```python
from build123d import *

# Parameters (mm, degrees)
F0_W     = 31.75
F0_H     = 88.9
F1_DEPTH = 2.54
F2_W     = 27.860178
F2_H     = 10.831637
F3_DEPTH = 25.4
F4_R     = 9.525
F5_DEPTH = 76.2
F6_R     = 7.62


with BuildPart() as f1:
    # F0 (on Top) → F1 (new body)
    with BuildSketch(Plane.XY):
        Rectangle(F0_W, F0_H)
    extrude(amount=F1_DEPTH)

    # F2 (on face) → F3 (join)
    with BuildSketch(Plane.XY.offset(2.54)):
        Polygon((15.875, -44.45), (15.875, 44.45), (14.305094, 44.45), (14.305094, -24.071639), (-13.428997, -24.071639), (-13.428997, 44.45), (-15.643887, 44.45), (-15.875, 44.45), (-15.875, -44.45), align=None)
        with Locations((0.375005, -33.933696)):
            Rectangle(F2_W, F2_H, mode=Mode.SUBTRACT)
    extrude(amount=F3_DEPTH)

    # F4 (on face) → F5 (join)
    with BuildSketch(Plane(origin=(0, -24.071639, 0), x_dir=(-1, 0, 0), z_dir=(0, 1, 0))):
        with Locations((0, 15.24)):
            Circle(F4_R)
    extrude(amount=F5_DEPTH)

    # F6
    f6_edges = [f1.edges().sort_by_distance(p)[0] for p in [
        (9.525, 52.128361, 15.24),
    ]]
    fillet(f6_edges, radius=F6_R)


solid = f1.part
```
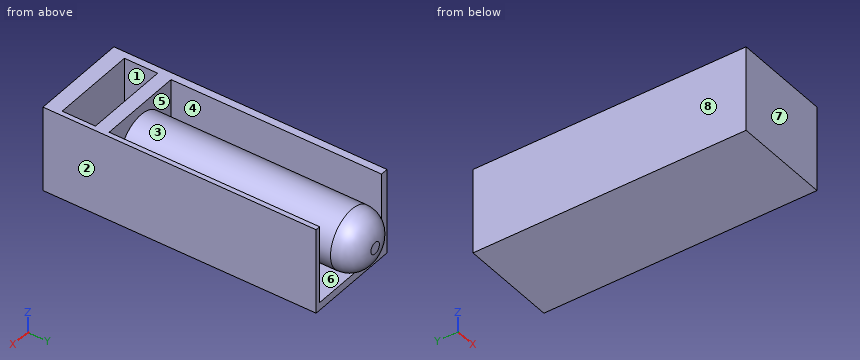
The model under review builds one solid part; all positions refer to its coordinate system, in mm. Face numbers are marked on the shaded views. A direction names the side the tool comes from. Give positions to 0.01 mm unless a question says otherwise; leave off trailing zeros. Loops run counter-clockwise (first coordinate to the right, second up) from the corner with the lowest first, then second, coordinate; pieces in that order, holes last. Notation, with made-up numbers: (63, 59.5) -> (74, 59.5) arc R30 cw to (74, 90.5) -> close; hole circle Ø11 at (1.25, 1). An arc over 180 degrees is marked (long way). Use CSV: the item, a comma, the result in double quotes.
1. Consider section B-B, the plane x = 11. Write out the cut boundary in (y, z).
Result:
outline,"(-44.45, 0) -> (44.45, 0) -> (44.45, 2.54) -> (-24.07, 2.54) -> (-24.07, 27.94) -> (-28.52, 27.94) -> (-28.52, 2.54) -> (-39.35, 2.54) -> (-39.35, 27.94) -> (-44.45, 27.94) -> close"
2. Consider section A-A, the plane y = -13. Write out the cut boundary in (x, z) (3 decimals).
Result:
outline,"(-15.875, 0) -> (15.875, 0) -> (15.875, 27.94) -> (14.305, 27.94) -> (14.305, 2.54) -> (-13.429, 2.54) -> (-13.429, 27.94) -> (-15.875, 27.94) -> close; circle Ø19.05 at (0, 15.24)"
3. To check wall thickness, follow probe 1 along Y at (x, z) = (-6, 7.5); probe 2 along X at (y, z) = (-38, 5) (3 decimals); probe 3 along X at (y, z) = (-15.5, 20.75) (3 decimals). State the ranges of each line that lie inside material, in increasing order. Write a range as from..to.
Result:
probe 1,"y = -44.45..-39.35, -28.52..-24.07"
probe 2,"x = -15.875..-13.555, 14.305..15.875"
probe 3,"x = -15.875..-13.429, -7.77..7.77, 14.305..15.875"
4. The part is to be moulded in two halves that separate along X. For the marked faces 5, 6, 7 and 8, say which applies: +X half, -X half, draft (parallel to the pull), parting line (faces both ways), or undercut.
Result:
face 5,"undercut"
face 6,"undercut"
face 7,"draft"
face 8,"-X half"
5. Consider section C-C, the plane z = 25.75. Write out the cut boundary in (x, y) (3 decimals), then the cut area to 3 significant figures.
Result:
outline,"(-15.875, -44.45) -> (15.875, -44.45) -> (15.875, 44.45) -> (14.305, 44.45) -> (14.305, -24.072) -> (-13.429, -24.072) -> (-13.429, 44.45) -> (-15.875, 44.45) -> close; hole (-13.555, -39.35) -> (14.305, -39.35) -> (14.305, -28.518) -> (-13.555, -28.518) -> close"
area,"620 mm²"
6. For P1, Ø12.5, axis at x = 4.5, z = 16, coming from the +Y side; P2, Ø8.5, axis at x = -0.5, y = 20, coming from the +Z side (3 decimals); P3, Ø1, axis at x = 5.5, z = 18.5, coming from the +Y side, all flat-tipped, find the tip position at first contact; note any pin that passes through.
Result:
P1,"stops at y = 52.13"
P2,"stops at z = 24.765"
P3,"stops at y = 51"
7. Machinability: for the marked faces 1, 2, 3 and 4, which of the approach directions +Z, -Z, +X, -X, +Y, -Y give a long, thin tool a straight path to every point of the face, cutting with its end or side? Answer none if there is none.
Result:
face 1,"+Z"
face 2,"+Z, -Z, +X, +Y, -Y"
face 3,"+Y"
face 4,"+Z, +Y"
8. Consider section D-D, the plane y = -32. Write out the cut boundary in (x, z) (3 decimals), then the cut area to 3 significant figures.
Result:
outline,"(-15.875, 0) -> (15.875, 0) -> (15.875, 27.94) -> (14.305, 27.94) -> (14.305, 2.54) -> (-13.555, 2.54) -> (-13.555, 27.94) -> (-15.875, 27.94) -> close"
area,"179 mm²"
